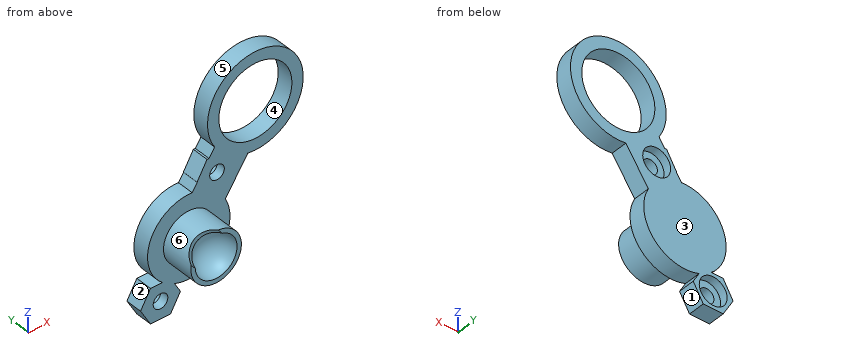
```python
from build123d import *

# Parameters (mm, degrees)
RETAINER_FEATURE_1_PROFILE_R  = 3.8
RETAINER_FEATURE_1_DEPTH      = 5.02
RETAINER_FEATURE_2_PROFILE_R  = 6.2
RETAINER_FEATURE_2_DEPTH      = 2.5
RETAINER_FEATURE_5_DEPTH      = 2.5
RETAINER_FEATURE_8_DEPTH      = 2.5
RETAINER_FEATURE_12_DEPTH     = 2.5
RETAINER_FEATURE_13_PROFILE_R = 7.2
RETAINER_FEATURE_13_DEPTH     = 2.5
RETAINER_FEATURE_14_PROFILE_R = 5.5
RETAINER_FEATURE_14_DEPTH     = 2.7
RETAINER_FEATURE_15_PROFILE_R = 1.1
RETAINER_FEATURE_15_DEPTH     = 3.75
RETAINER_FEATURE_16_PROFILE_R = 2.1
RETAINER_FEATURE_16_DEPTH     = 1.45
RETAINER_FEATURE_17_PROFILE_R = 1.1
RETAINER_FEATURE_17_DEPTH     = 3.75
RETAINER_FEATURE_18_PROFILE_R = 2.1
RETAINER_FEATURE_18_DEPTH     = 1.45


with BuildPart() as part:
    # Retainer Feature 1 profile → Retainer Feature 1 (new body)
    with BuildSketch(Plane(origin=(0, -101, 0), x_dir=(-1, 0, 0), z_dir=(0, -1, 0))):
        with Locations(Location((30.310889132, 15, 0), (0, 0, 90))):
            Circle(RETAINER_FEATURE_1_PROFILE_R)
    extrude(amount=RETAINER_FEATURE_1_DEPTH)

    # Retainer Feature 2 profile → Retainer Feature 2 (add)
    with BuildSketch(Plane(origin=(0, -106, 0), x_dir=(-1, 0, 0), z_dir=(0, -1, 0))):
        with Locations(Location((30.310889132, 15, 0), (0, 0, 90))):
            Circle(RETAINER_FEATURE_2_PROFILE_R)
    extrude(amount=RETAINER_FEATURE_2_DEPTH)

    # Middle Right Floating Compression Ball R → Retainer Feature 5 (add)
    with BuildSketch(Plane(origin=(0, -106, 0), x_dir=(-1, 0, 0), z_dir=(0, -1, 0))):
        Polygon((31.560889132, 22.361215932), (33.060889132, 19.763139721), (36.060889132, 19.763139721), (37.560889132, 22.361215932), (36.060889132, 24.959292144), (33.060889132, 24.959292144), align=None)
    extrude(amount=RETAINER_FEATURE_5_DEPTH)

    # Middle Right Floating Compression Ba 2 → Retainer Feature 8 (add)
    with BuildSketch(Plane(origin=(0, -106, 0), x_dir=(-1, 0, 0), z_dir=(0, -1, 0))):
        Polygon((23.060889132, 7.638784068), (24.560889132, 5.040707856), (27.560889132, 5.040707856), (29.060889132, 7.638784068), (27.560889132, 10.236860279), (24.560889132, 10.236860279), align=None)
    extrude(amount=RETAINER_FEATURE_8_DEPTH)

    # Retainer Feature 9 profile → Retainer Feature 9 (revolve, cut)
    with BuildSketch(Plane(origin=(0, -101, 0), x_dir=(-1, 0, 0), z_dir=(0, -1, 0))):
        with BuildLine():
            Line((30.310889132, 11.85), (30.310889132, 18.15))
            ThreePointArc((30.310889132, 18.15), (27.160889132, 15), (30.310889132, 11.85))
        make_face()
    revolve(axis=Axis((-30.310889132, -101, -25), (0, 0, 1)), mode=Mode.SUBTRACT)

    # Middle Right Floating Compression Ba 3 → Retainer Feature 12 (add)
    with BuildSketch(Plane(origin=(0, -106, 0), x_dir=(-1, 0, 0), z_dir=(0, -1, 0))):
        Polygon((27.816215917, 16.66631496), (17.79697803, 1.66631496), (22.786324462, -1.66631496), (32.805562348, 13.33368504), align=None)
    extrude(amount=RETAINER_FEATURE_12_DEPTH)

    # Retainer Feature 13 profile → Retainer Feature 13 (add)
    with BuildSketch(Plane(origin=(0, -106, 0), x_dir=(-1, 0, 0), z_dir=(0, -1, 0))):
        with Locations((20.291651246, 0)):
            Circle(RETAINER_FEATURE_13_PROFILE_R)
    extrude(amount=RETAINER_FEATURE_13_DEPTH)

    # Retainer Feature 14 profile → Retainer Feature 14 (cut)
    with BuildSketch(Plane(origin=(0, -105.9, 0), x_dir=(-1, 0, 0), z_dir=(0, -1, 0))):
        with Locations(Location((20.291651246, 0, 0), (0, 0, 270))):
            Circle(RETAINER_FEATURE_14_PROFILE_R)
    extrude(amount=RETAINER_FEATURE_14_DEPTH, mode=Mode.SUBTRACT)

    # Retainer Feature 15 profile → Retainer Feature 15 (cut)
    with BuildSketch(Plane(origin=(0, -105, 0), x_dir=(-1, 0, 0), z_dir=(0, -1, 0))):
        with Locations(Location((34.560889132, 22.361215932, 0), (0, 0, 90))):
            Circle(RETAINER_FEATURE_15_PROFILE_R)
    extrude(amount=RETAINER_FEATURE_15_DEPTH, mode=Mode.SUBTRACT)

    # Retainer Feature 16 profile → Retainer Feature 16 (cut)
    with BuildSketch(Plane(origin=(0, -107.3, 0), x_dir=(-1, 0, 0), z_dir=(0, -1, 0))):
        with Locations(Location((34.560889132, 22.361215932, 0), (0, 0, 90))):
            Circle(RETAINER_FEATURE_16_PROFILE_R)
    extrude(amount=RETAINER_FEATURE_16_DEPTH, mode=Mode.SUBTRACT)

    # Retainer Feature 17 profile → Retainer Feature 17 (cut)
    with BuildSketch(Plane(origin=(0, -105, 0), x_dir=(-1, 0, 0), z_dir=(0, -1, 0))):
        with Locations(Location((26.060889132, 7.638784068, 0), (0, 0, 90))):
            Circle(RETAINER_FEATURE_17_PROFILE_R)
    extrude(amount=RETAINER_FEATURE_17_DEPTH, mode=Mode.SUBTRACT)

    # Retainer Feature 18 profile → Retainer Feature 18 (cut)
    with BuildSketch(Plane(origin=(0, -107.3, 0), x_dir=(-1, 0, 0), z_dir=(0, -1, 0))):
        with Locations(Location((26.060889132, 7.638784068, 0), (0, 0, 90))):
            Circle(RETAINER_FEATURE_18_PROFILE_R)
    extrude(amount=RETAINER_FEATURE_18_DEPTH, mode=Mode.SUBTRACT)

    # Articulation Throat Sketch → Articulation Throat (revolve, cut)
    with BuildSketch(Plane(origin=(-55.559435073, -21.315405316, -26.260716517), x_dir=(0.37694407644157146, 0.1446147852349051, -0.9148768917876727), z_dir=(0.8541721659092646, 0.32770358269776195, 0.4037329227012915))):
        Polygon((-12.308450042, -83.441173866), (-10.724100051, -81.773890115), (-22.767880189, -61.059022025), (-28.981287547, -67.597673951), align=None)
    revolve(axis=Axis((-25.110986143, -106.383086561, -21.631997284), (-0.5199902989343897, 0.5383086561091633, 0.6631997284167648)), mode=Mode.SUBTRACT)


with BuildPart() as body_2:
    # Mirror1: mirrored copy
    add(part.part.mirror(Plane(origin=(0, 0, 0), x_dir=(0, 0, 1), z_dir=(0, -1, 0))))


solid = body_2.part
```
Model file for the job. Use its own axes, mm. Face numbers are marked on the shaded views. A direction names the side the tool comes from. Coordinates: 2 decimals unless noted, no trailing zeros. Order: outer loops, then holes, each group sorted by start corner. A loop starts at its lowest first (then second) coordinate and runs counter-clockwise, first axis right, second up. Notation, with made-up numbers: (34.25, -16) - (39.25, -16) arc R25 ccw to (39.25, 3) - close; hole circle Ø8 at (59, -1.75). An arc over 180 degrees is marked (long way). Return JSON: item names as keys, results as strings. Group by question number.
1) Tool access for the marked faces 5 and 6: list every direction of +Z, -Z, +X, -X, +Y, -Y with a clear straight run to the whole face (end or side of a thin tool).
2) Saw through at A-A, the plane z = 0. Write the cut outline in (x, y), plus the area to 3 significant figures.
3) Saw through at B-B, the plane y = 103.75. Write the cut outline in (x, z), plus the area to 3 significant figures.
4) Probe line 1 (Y direction, x = -30.75, z = -10.5); line 2 (X direction, y = 102.75, z = -14); line 3 (X direction, y = 106.5, z = 2) (3 decimals). List the from-to ranges inside material, lowest first. Write a range as from..to.
5) Flat gauge pins, fed straight in: P1, Ø2, axis at x = -32.5, z = -10.5, coming from the -Y side; P2, Ø2.5, axis at x = -26.06, z = -7.64, coming from the +Y side; P3, Ø2, axis at x = -35.5, y = 107, coming from the +Z side. Where does each tip first touch, or does it go through?
6) Mould opens along X. For the marked faces 1, 2, 3 and 4 say: released by +X, released by -X, zero draft, split by the parting line, or undercut.
Values found:
{
 "1": {"face 5": "+Y, -Y", "face 6": "-Y"},
 "2": {"outline": "(-27.49, 106) - (-25.79, 106) - (-25.79, 108.5) - (-27.49, 108.5) - close; (-14.79, 106) - (-13.09, 106) - (-13.09, 108.5) - (-14.79, 108.5) - close", "area": "8.50 mm²"},
 "3": {"outline": "circle Ø7.6 at (-30.31, -15); hole circle Ø3.07 at (-30.31, -15)", "area": "38.0 mm²"},
 "4": {"line 1": "y = 106..108.5", "line 2": "x = -33.98..-32.73, -27.89..-26.64", "line 3": "x = -27.208..-25.415, -15.168..-13.375"},
 "5": {"P1": "stops at y = 106", "P2": "stops at y = 107.3", "P3": "stops at z = -10.43"},
 "6": {"face 1": "released by +X", "face 2": "released by -X", "face 3": "zero draft", "face 4": "undercut"}
}
